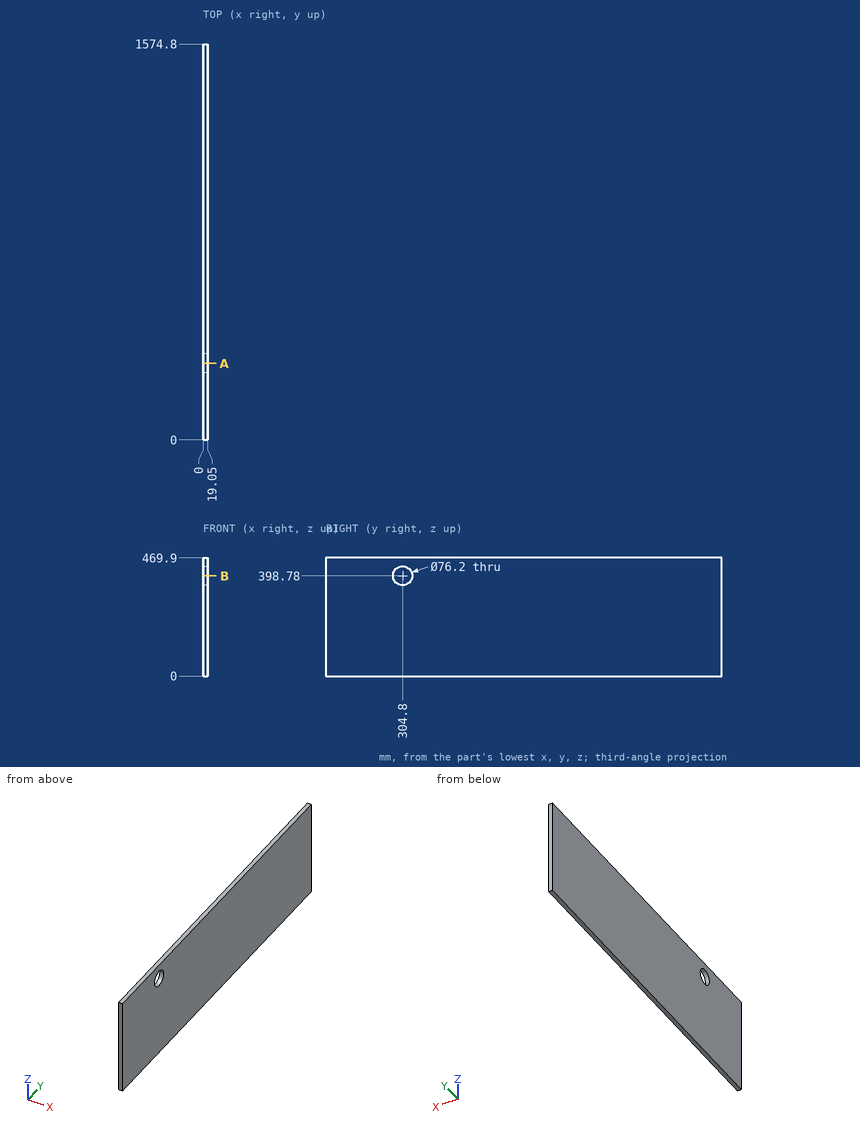
Input: dimensioned drawing with shaded views. Units: mm. Origin: part minimum x, y, z. Coordinates: 2 decimals unless noted, no trailing zeros. Loops run counter-clockwise (first coordinate to the right, second up) from the corner with the lowest first, then second, coordinate; pieces in that order, holes last. Notation, with made-up numbers: M 59,52 L 76,52 A18 ccw 76,65 Z; hole C -1,43.25 d9. An arc over 180 degrees is marked long. One line per item, written item: value. Start each with the question number.
1) Pin query (flat end, axial travel): P1, Ø5, axis at x = 8, y = 966.5, coming from the -Z side. Return the tip coordinate at first contact, or that it passes through.
2) Cut plane A-A (y = 304.8). Return loops of the section in (x, z), then the cut area to 3 significant figures.
3) Material intervals for L1, parallel to Y at x = 14.25, z = 398.78; L2, parallel to Y at x = 4.5, z = 416, sorted ascending. Write a range as from..to.
4) Cut plane B-B (z = 398.78). Return loops of the section in (x, y), then the cut area to 3 significant figures.
Evaluation:
1. P1: z = 0
2. outline: M 0,0 L 19.05,0 L 19.05,360.68 L 0,360.68 Z; M 0,436.88 L 19.05,436.88 L 19.05,469.9 L 0,469.9 Z
2. area: 7,500 mm^2
3. L1: 0..266.7, 342.9..1574.8
3. L2: 0..270.81, 338.79..1574.8
4. outline: M 0,0 L 19.05,0 L 19.05,266.7 L 0,266.7 Z; M 0,342.9 L 19.05,342.9 L 19.05,1574.8 L 0,1574.8 Z
4. area: 28,500 mm^2
